Geometry check sheet. Reference: drawing and pictorial views, mm from the part's lowest x, y, z. Give positions to 0.01 mm unless a question says otherwise; leave off trailing zeros. Write each loop counter-clockwise with the first axis right and the second up, starting at its lowest first coordinate (ties: lowest second). Pieces come first, ordered by that corner, then holes. Notation, with made-up numbers: (71.5, 55) -> (107.5, 55) arc R24 cw to (107.5, 93) -> close; hole circle Ø7 at (-24.75, -9.75). An arc over 180 degrees is marked (long way). Write each question's results on one line, items separated by ' | '. Start each with the question number.
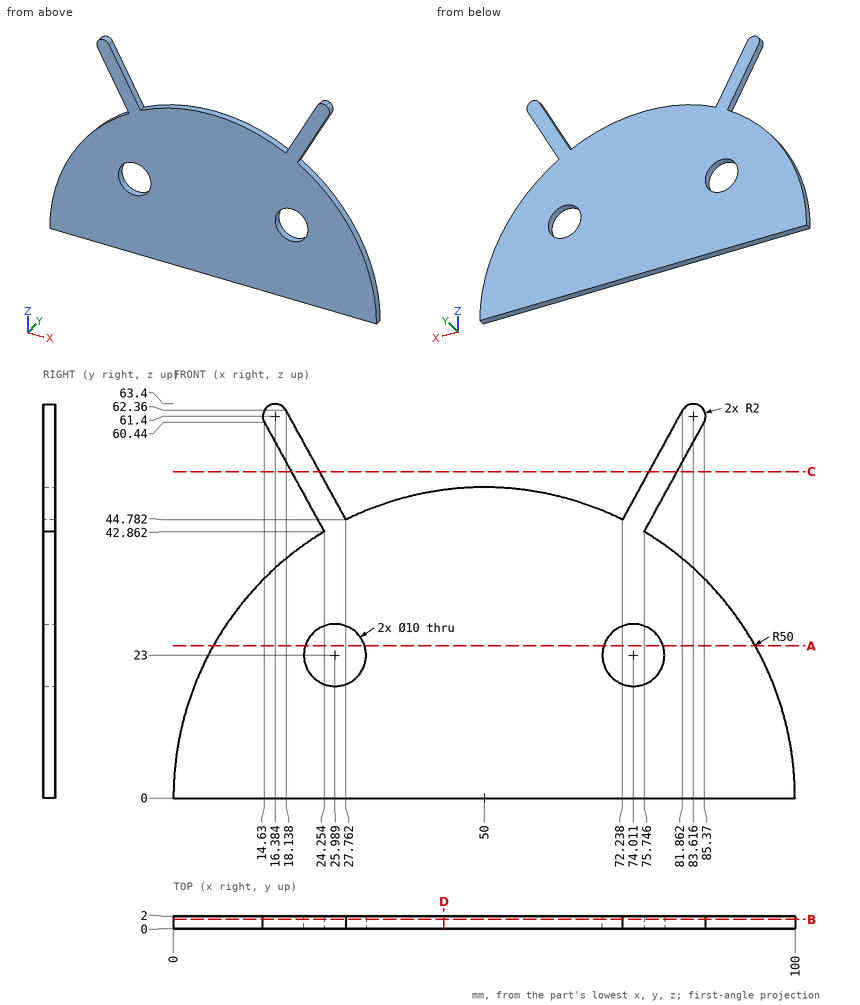
Item 1: Section check B-B on y = 1.45. Record the boundary of the cut face in (x, z) (1 decimal).
Item 2: Thickness scan on probe 1 along X at (y, z) = (0.15, 26.5); probe 2 along X at (y, z) = (0.4, 21) (1 decimal); probe 3 along Z at (x, y) = (78, 0.3) (1 decimal). Record the ranges inside material, lowest first. Write a range as from..to.
Item 3: Section check D-D on x = 43.5. Record the boundary of the cut face in (y, z) (1 decimal).
Item 4: Section check A-A on z = 24.5. Record the boundary of the cut face in (x, y).
Item 5: Section check C-C on z = 52.5. Record the boundary of the cut face in (x, y).
Item 6: Depth check by flat-ended pin: pin 1 Ø16 at (x, z) = (74.01, 23) entering from +Y; pin 2 Ø1 at (y, z) = (0.5, 31.5) entering from +X. Enter the tip coordinate at first touch or a pass-through.
Check sheet entries:
1) outline: (0, 0) -> (100, 0) arc R50 ccw to (75.7, 42.9) -> (85.4, 60.4) arc R2 ccw to (84.6, 63.2) arc R2 ccw to (81.9, 62.4) -> (72.2, 44.8) arc R50 ccw to (27.8, 44.8) -> (18.1, 62.4) arc R2 ccw to (15.4, 63.2) arc R2 ccw to (14.6, 60.4) -> (24.3, 42.9) arc R50 ccw to start; hole circle Ø10 at (26, 23); hole circle Ø10 at (74, 23)
2) probe 1: x = 7.6..22.42, 29.56..70.44, 77.58..92.4 | probe 2: x = 4.6..21.4, 30.6..69.4, 78.6..95.4 | probe 3: z = 0..20, 26..41.4, 47..55.3
3) outline: (0, 0) -> (2, 0) -> (2, 49.6) -> (0, 49.6) -> close
4) outline: (6.41, 0) -> (21.22, 0) -> (21.22, 2) -> (6.41, 2) -> close; (30.76, 0) -> (69.24, 0) -> (69.24, 2) -> (30.76, 2) -> close; (78.78, 0) -> (93.59, 0) -> (93.59, 2) -> (78.78, 2) -> close
5) outline: (18.98, 0) -> (23.54, 0) -> (23.54, 2) -> (18.98, 2) -> close; (76.46, 0) -> (81.02, 0) -> (81.02, 2) -> (76.46, 2) -> close
6) pin 1: stops at y = 2 | pin 2: stops at x = 89.23
